Work out the finished part from the listing and answer in its coordinate system (mm). Give positions to 0.01 mm unless a question says otherwise; leave off trailing zeros. Loops run counter-clockwise (first coordinate to the right, second up) from the corner with the lowest first, then second, coordinate; pieces in that order, holes last. Notation, with made-up numbers: (-27.75, 77) - (30.25, 77) arc R18 ccw to (30.25, 83) - close; hole circle Ø8 at (33, 60.25). An arc over 180 degrees is marked (long way). Use CSV: the item, a comma, the result in double quotes.
Autodesk Inventor part; units mm, degrees
ref_plane "YZ Plane" through (0, 0, 0) normal (1, 0, 0) x (0, 1, 0)
ref_plane "XZ Plane" through (0, 0, 0) normal (0, 1, 0) x (-1, 0, 0)
ref_plane "XY Plane" through (0, 0, 0) normal (0, 0, 1) x (1, 0, 0)
ref_plane "Work Plane1" through (0, 0, 0) normal (0, 0, 1) x (1, 0, 0)
sketch "Sketch1" plane through (0, 0, 0) normal (0, 0, 1) x (1, 0, 0)
  circle A0 centre (-29.8289, -24.3423) radius 1.1
  point P0 (0, 0)
extrude "Extrusion1" add sketch "Sketch1" against normal blind 6.35
ref_plane "Work Plane2" through (0, 0, 0) normal (0, 0, 1) x (1, 0, 0)
sketch "Sketch2" plane through (0, 0, 0) normal (0, 0, 1) x (1, 0, 0)
  circle A0 centre (-29.8289, -24.3423) radius 1.1
  circle A1 centre (-29.8289, -24.3423) radius 2.25
  point P0 (0, 0)
  dimension "d5" = 4.5
extrude "Extrusion3" add sketch "Sketch2" along normal blind 20 contours A0 | A1
sketch "Sketch3" plane through (-29.8289, -24.3423, 20) normal (0, 0, 1) x (1, 0, 0)
  circle A0 centre (0, 0) radius 1.1
  point P0 (29.8289, 24.3423)
extrude "Extrusion4" cut sketch "Sketch3" against normal blind 6.35
properties part number "standoff" material "Stainless Steel"
Item 1: A cutting plane is placed at D-D on z = -3.75. Determine the outline of the cut face in (x, y).
Determined:
outline,"circle Ø2.2 at (-29.83, -24.34)"
Item 2: Find the intervals of material crossed by line 1 (Z direction, x = -29.25, y = -25.1); line 2 (Z direction, x = -29.4, y = -26.2); line 3 (Y direction, x = -29.35, z = 17), in increasing order.
Determined:
line 1,"z = -6.35 to 13.65"
line 2,"z = 0 to 20"
line 3,"y = -26.54 to -25.33, -23.35 to -22.14"
Item 3: A cutting plane is placed at C-C on z = 15.5. Determine the outline of the cut face in (x, y).
Determined:
outline,"circle Ø4.5 at (-29.83, -24.34); hole circle Ø2.2 at (-29.83, -24.34)"
Item 4: The mould has two halves that part along Y. Classify faces 1 (the cylindrical face through (-28.81, -24.76, -3.13)), 2 (the cylindrical face through (-28.81, -24.76, 16.87)), 3 (the flat face through (-30, -24, 13.65)), 4 (the flat face through (-29, -23, 0)): pulls with the +Y half, pulls with the -Y half, needs draft (parallel to the pull), parting line crosses it, or undercut.
Determined:
face 1,"parting line crosses it"
face 2,"undercut"
face 3,"undercut"
face 4,"needs draft"
Item 5: Given P1, Ø1.5, axis at x = -31, z = 13.5, coming from the +Y side; P2, Ø1.1, axis at x = -30, y = -24.5, coming from the +Z side, each flat-ended and moving along its own axis, determine where each tip first touches the part or whether it passes through.
Determined:
P1,"stops at y = -22.13"
P2,"stops at z = 13.65"
Item 6: A cutting plane is placed at B-B on y = -24.1. Determine the outline of the cut face in (x, z).
Determined:
outline,"(-32.07, 0) - (-30.9, 0) - (-30.9, -6.35) - (-28.76, -6.35) - (-28.76, 0) - (-27.59, 0) - (-27.59, 20) - (-28.76, 20) - (-28.76, 13.65) - (-30.9, 13.65) - (-30.9, 20) - (-32.07, 20) - close"
Item 7: A cutting plane is placed at A-A on x = -29.4. Determine the outline of the cut face in (y, z), and give its area (3 significant figures).
Determined:
outline,"(-26.55, 0) - (-25.36, 0) - (-25.36, -6.35) - (-23.33, -6.35) - (-23.33, 0) - (-22.13, 0) - (-22.13, 20) - (-23.33, 20) - (-23.33, 13.65) - (-25.36, 13.65) - (-25.36, 20) - (-26.55, 20) - close"
area,"88.3 mm²"
